Autodesk Inventor part; units mm, degrees
ref_plane "YZ Plane" through (0, 0, 0) normal (1, 0, 0) x (0, 1, 0)
ref_plane "XZ Plane" through (0, 0, 0) normal (0, 1, 0) x (-1, 0, 0)
ref_plane "XY Plane" through (0, 0, 0) normal (0, 0, 1) x (1, 0, 0)
sketch "Sketch1" plane through (0, 0, 0) normal (0, 0, 1) x (1, 0, 0)
  line L0 (96, 0) -> (0, 0)
  line L1 (0, 0) -> (0, 24)
  line L2 (0, 24) -> (96, 24)
  line L3 (96, 24) -> (96, 0)
  point P0 (0, 0)
  dimension "d0" = 96
  dimension "d1" = 24
extrude "Extrusion1" add sketch "Sketch1" along normal blind 8
sketch "Sketch5" plane through (0, 0, 8) normal (0, 0, 1) x (1, 0, 0)
  circle A0 centre (88, 20) radius 2.5
  line L0 (144, 20) -> (0, 20) construction
  line L1 (88, 24) -> (88, 0) construction
  line L2 (96, 24) -> (0, 24) construction
  line L3 (0, 0) -> (96, 0) construction
  line L4 (0, 24) -> (96, 24) construction
  line L5 (96, 24) -> (96, 0) construction
  line L6 (96, 0) -> (0, 0) construction
  line L7 (0, 0) -> (0, 24) construction
  circle A1 centre (72, 20) radius 2.5
  circle A2 centre (56, 20) radius 2.5
  circle A3 centre (40, 20) radius 2.5
  circle A4 centre (24, 20) radius 2.5
  circle A5 centre (8, 20) radius 2.5
  circle A6 centre (88, 4) radius 2.5
  circle A7 centre (72, 4) radius 2.5
  circle A8 centre (56, 4) radius 2.5
  circle A9 centre (40, 4) radius 2.5
  circle A10 centre (24, 4) radius 2.5
  circle A11 centre (8, 4) radius 2.5
  dimension "d30" = 5
  dimension "d83" = 4
  dimension "d84" = 8
  dimension "d87" = 16
  dimension "d90" = 16
extrude "Extrusion8" cut sketch "Sketch5" against normal through all
sketch "Sketch9" plane through (96, 0, 0) normal (1, 0, 0) x (0, 0, -1)
  circle A0 centre (-4, 20) radius 2
  circle A1 centre (-4, 4) radius 2
  line L0 (0, 0) -> (-8, 0)
  line L1 (0, 24) -> (-8, 24) construction
  line L2 (-8, 24) -> (0, 24) construction
  line L3 (0, 24) -> (0, 0) construction
  line L4 (0, 0) -> (-8, 0) construction
  line L5 (-8, 0) -> (-8, 24) construction
  point P0 (0, 0)
  dimension "d95" = 4
  dimension "d96" = 4
  dimension "d97" = 4
  dimension "d98" = 4
  dimension "d99" = 4
  dimension "d100" = 4
extrude "Extrusion9" cut sketch "Sketch9" against normal blind 4
sketch "Sketch10" plane through (0, 0, 0) normal (-1, 0, 0) x (0, 0, 1)
  line L0 (0, 24) -> (0, 0) construction
  line L1 (0, 24) -> (8, 24) construction
  line L2 (8, 24) -> (8, 0) construction
  line L3 (8, 0) -> (0, 0) construction
  line L4 (0, 0) -> (0, 24) construction
  circle A0 centre (4, 20) radius 2
  circle A1 centre (4, 4) radius 2
  point P0 (0, 0)
  dimension "d107" = 4
  dimension "d108" = 4
  dimension "d109" = 4
  dimension "d110" = 4
  dimension "d111" = 4
  dimension "d112" = 4
extrude "Extrusion10" cut sketch "Sketch10" against normal blind 4
sketch "Sketch11" plane through (0, 0, 0) normal (0, 0, -1) x (-1, 0, 0)
  line L0 (-96, 24) -> (-96, 0)
  line L1 (-96, 14) -> (48, 14)
  line L2 (48, 14) -> (48, 10)
  line L3 (48, 10) -> (-96, 10)
  line L4 (-96, 10) -> (-96, 14)
  line L5 (0, 24) -> (-96, 24)
  line L6 (-96, 0) -> (0, 0)
  point P0 (0, 0)
  dimension "d119" = 10
  dimension "d120" = 10
  dimension "d121" = 144
extrude "Extrusion11" cut sketch "Sketch11" against normal blind 6
properties part number "Beam0824-096-Blue" material "Aluminum 6061"
The model under review builds one solid part; all positions refer to its coordinate system, in mm. A direction names the side the tool comes from. Round coordinates to 2 decimals unless told otherwise and drop trailing zeros. Order: outer loops, then holes, each group sorted by start corner. A loop starts at its lowest first (then second) coordinate and runs counter-clockwise, first axis right, second up. Notation, with made-up numbers: (44, -38.75) -> (87, -38.75) arc R20 ccw to (87, -29.75) -> close; hole circle Ø1 at (53, -8). An arc over 180 degrees is marked (long way). One line per item, written item: value. Start each with the question number.
Q1. Clearance check with flat-ended pins moving along their axes: pin 1 Ø2.5 at (y, z) = (4, 4) entering from +X; pin 2 Ø1.2 at (y, z) = (3.5, 4.5) entering from -X. State where each tip first meets the part, or that it passes through.
Q2. Take a section at B-B (x = 72). Write out the cut boundary in (y, z).
Q3. Machinability: for faces 1 (the face through (42.31, 3.04, 4.06)), 2 (the face through (47, 10, 3)), 3 (the face through (92, 20, 4)), 4 (the face through (4, 20, 4)), which of the approach directions +Z, -Z, +X, -X, +Y, -Y give a long, thin tool a straight path to every point of the face, cutting with its end or side? Answer none if there is none.
Q4. Wall thickness on line 1 (Y direction, x = 88, z = 5); line 2 (Y direction, x = 88, z = 7.75); line 3 (Y direction, x = 31, z = 1.25): over which ranges is each line inside the solid? List them lowest first.
Q5. Take a section at A-A (z = 1). Count the separate pieces of the cut face and the enclosed holes in it, and give its area (3 significant figures).
Q6. Take a section at D-D (x = 49.5). Write out the cut boundary in (y, z), and give its area (3 significant figures).
Q7. Mouldability with a two-part tool opening along Y and no side actions: class faces 5 (the face through (96, 12, 7)), 6 (the face through (49, 0, 4)), 7 (the face through (23.67, 22.48, 4.06)) as released by +Y, released by -Y, zero draft, split by the parting line, or undercut.
Reported:
1. pin 1: stops at x = 92
1. pin 2: stops at x = 4
2. outline: (0, 0) -> (1.5, 0) -> (1.5, 8) -> (0, 8) -> close; (6.5, 0) -> (10, 0) -> (10, 6) -> (14, 6) -> (14, 0) -> (17.5, 0) -> (17.5, 8) -> (6.5, 8) -> close; (22.5, 0) -> (24, 0) -> (24, 8) -> (22.5, 8) -> close
3. face 1: +Z, -Z
3. face 2: -Z, +X, -X
3. face 3: +X
3. face 4: -X
4. line 1: y = 0 to 1.5, 6.5 to 10, 14 to 17.5, 22.5 to 24
4. line 2: y = 0 to 1.5, 6.5 to 17.5, 22.5 to 24
4. line 3: y = 0 to 10, 14 to 24
5. separate pieces: 2
5. enclosed holes: 12
5. area: 1,680 mm2
6. outline: (0, 0) -> (10, 0) -> (10, 6) -> (14, 6) -> (14, 0) -> (24, 0) -> (24, 8) -> (0, 8) -> close
6. area: 168 mm2
7. face 5: zero draft
7. face 6: released by -Y
7. face 7: undercut
